Geometry check sheet. Reference: the model listing, model coordinates, mm. A direction names the side the tool comes from. Round coordinates to 2 decimals unless told otherwise and drop trailing zeros. Write each loop counter-clockwise with the first axis right and the second up, starting at its lowest first coordinate (ties: lowest second). Pieces come first, ordered by that corner, then holes. Notation, with made-up numbers: M 28,9.25 L 87,9.25 A24 cw 87,43.25 Z; hole C -27.75,84.5 d8. An arc over 180 degrees is marked long. Put each result on its own line as item: value. Start each with the question number.
(1) Section check B-B on y = -5.5. Record the cut outline in (x, z).
(2) Section check A-A on y = 1.25. Record the cut outline in (x, z), then the cut area to 3 significant figures.
(3) Tool access check on faces 1 (the conical face through (-0.2, -0.7, -8.92)), 2 (the cylindrical face through (-0.259, 6.108, -11.797)), 3 (the cylindrical face through (-0.1, -10.2, -6.8)). Record the directions out of +Z, -Z, +X, -X, +Y, -Y that give a thin tool (end or side, any length) a straight path to the whole face; none if there is none.
(4) Material ranges on probe 1 along Y at (x, z) = (-11, -1.25); probe 2 along X at (y, z) = (2, -4.5); probe 3 along X at (y, z) = (-2, -4.75), recorded low to high.
(5) Mould release check, pull along Y, two halves, no side actions. Record for faces 4 (the flat face through (0, 6.65, -12)), 5 (the conical face through (-0.2, 3.1, -10.8)), 6 (the conical face through (-0.13, -8.31, -5.76)): pulls with the +Y half, pulls with the -Y half, needs draft (parallel to the pull), parting line crosses it, or undercut.
(6) Gauge pin test, flat ends, axial feed: pin 1 (10 mm diameter, centred on x = 7, y = 2, fed in from -Z); pin 2 (6 mm diameter, centred on y = -6.5, z = -6.5, fed in from +X); pin 3 (1 mm diameter, centred on y = 1.5, z = -8, fed in from +X). Record the tip position at first contact, or that the pin passes through.
from build123d import *

# Parameters (mm, degrees)
F1_ANGLE     = 180
F2_T4_ANGLE  = 243.2500896942
F2_S5_R      = 11.8
F2_T6_DEPTH  = 16
F3_T4_ANGLE  = 243.6352501502
F3_S5_R      = 11.8
F3_T6_DEPTH  = 16
F4_T4_ANGLE  = 309.1355997924
F4_S5_R      = 6.8
F4_T6_DEPTH  = 11
F4_T10_ANGLE = 243.2500896942
F4_S11_R     = 11.8
F4_T12_DEPTH = 16
F5_SIZE      = 0.75
F6_SIZE      = 1


# Not quite as in the source:
# - a fillet or chamfer that OpenCascade refuses, or shapes differently, is made with other operations: its cross-section is extruded or revolved along the edge and cut away or added
# - a feature names something its author has since deleted; it is built from what else it names


with BuildPart() as f1:
    # F0 (on Top) → F1 (revolve)
    with BuildSketch(Plane.XY):
        Polygon((-11.8, 5.65), (-11.8, 6.65), (-13.8, 6.65), (-13.8, 0), (-7.8, -10.95), (-6.8, -10.95), (-6.8, -9.45), (-4.8, -9.45), (-4.8, -7.45), (-9.8, 1), (-11.8, 1), (-11.8, 2), (-9.8, 2), (-9.8, 5.65), align=None)
    revolve(axis=Axis((0, 0, 0), (0, -1, 0)), revolution_arc=F1_ANGLE)

    # F2: chamfer of 2.1 on 1 edges, made by hand


with BuildPart() as f2_tool2:
    # F2_s3 → F2_t4 (revolve)
    with BuildSketch(Plane(origin=(0, 0, 0), x_dir=(0, 1, 0), z_dir=(0.5243581586, 0, 0.8514978107))):
        Polygon((3.55, 9.8), (5.65, 11.9), (5.65, 9.8), align=None)
    revolve(axis=Axis((0, 5.65, 0), (0, -1, 0)), revolution_arc=F2_T4_ANGLE)

    # F2_s5 → F2_t6 (intersect, symmetric)
    with BuildSketch(Plane.XZ.offset(-4.6)):
        Circle(F2_S5_R)
    extrude(amount=F2_T6_DEPTH, both=True, mode=Mode.INTERSECT)


with BuildPart() as f1_1:
    add(f1.part)

    # F2_t1: cut F2_tool2
    add(f2_tool2.part, mode=Mode.SUBTRACT)

    # F3: chamfer of 2.1 on 1 edges, made by hand


with BuildPart() as f3_tool2:
    # F3_s3 → F3_t4 (revolve)
    with BuildSketch(Plane(origin=(0, 0, 0), x_dir=(0, 1, 0), z_dir=(0.5272172108, 0, 0.849730553))):
        Polygon((-0.8073066866, 8.7305877594), (1, 11.9), (1, 9.8), align=None)
    revolve(axis=Axis((0, 1, 0), (0, -1, 0)), revolution_arc=F3_T4_ANGLE)

    # F3_s5 → F3_t6 (intersect, symmetric)
    with BuildSketch(Plane.XZ.offset(-0.1)):
        Circle(F3_S5_R)
    extrude(amount=F3_T6_DEPTH, both=True, mode=Mode.INTERSECT)


with BuildPart() as f1_2:
    add(f1_1.part)

    # F3_t1: cut F3_tool2
    add(f3_tool2.part, mode=Mode.SUBTRACT)

    # F4: chamfer of 2.1 on 2 edges, made by hand


with BuildPart() as f4_tool2:
    # F4_s3 → F4_t4 (revolve)
    with BuildSketch(Plane(origin=(0, 0, 0), x_dir=(0, 1, 0), z_dir=(0.9030940896, 0, 0.4294427381))):
        Polygon((-7.35, 4.8), (-9.45, 6.9), (-9.45, 4.8), align=None)
    revolve(axis=Axis((0, -9.45, 0), (0, -1, 0)), revolution_arc=F4_T4_ANGLE)

    # F4_s5 → F4_t6 (intersect, symmetric)
    with BuildSketch(Plane.XZ.offset(8.4)):
        Circle(F4_S5_R)
    extrude(amount=F4_T6_DEPTH, both=True, mode=Mode.INTERSECT)


with BuildPart() as f1_3:
    add(f1_2.part)

    # F4_t1: cut F4_tool2
    add(f4_tool2.part, mode=Mode.SUBTRACT)


with BuildPart() as f4_tool8:
    # F4_s9 → F4_t10 (revolve)
    with BuildSketch(Plane(origin=(0, 0, 0), x_dir=(0, 1, 0), z_dir=(0.5243581586, 0, 0.8514978107))):
        Polygon((4.1, 9.8), (2, 11.9), (2, 9.8), align=None)
    revolve(axis=Axis((0, 2, 0), (0, -1, 0)), revolution_arc=F4_T10_ANGLE)

    # F4_s11 → F4_t12 (intersect, symmetric)
    with BuildSketch(Plane.XZ.offset(-3)):
        Circle(F4_S11_R)
    extrude(amount=F4_T12_DEPTH, both=True, mode=Mode.INTERSECT)


with BuildPart() as f1_4:
    add(f1_3.part)

    # F4_t7: cut F4_tool8
    add(f4_tool8.part, mode=Mode.SUBTRACT)

    # F5
    f5_edges = [f1_4.edges().sort_by_distance(p)[0] for p in [
        (0, 3.825, -10.075),
    ]]
    chamfer(f5_edges, length=F5_SIZE)

    # F6
    f6_edges = [f1_4.edges().sort_by_distance(p)[0] for p in [
        (0, -7.387175, -4.837175),
    ]]
    chamfer(f6_edges, length=F6_SIZE)


solid = f1_4.part
Answers follow:
1. outline: M -10.79,0 A10.79 ccw 10.79,0 L 5.95,0 A5.95 cw -5.95,0 Z
2. outline: M -13.8,0 A13.8 ccw 13.8,0 L 11.8,0 A11.8 cw -11.8,0 Z
2. area: 80.4 mm^2
3. face 1: +Z
3. face 2: +Z, +Y
3. face 3: +Z, -Y
4. probe 1: y = -4.98 to 0.53, 2.83 to 4.82
4. probe 2: x = -13.05 to -10.91, 10.91 to 13.05
4. probe 3: x = -11.78 to -6.47, 6.47 to 11.78
5. face 4: pulls with the +Y half
5. face 5: undercut
5. face 6: pulls with the -Y half
6. pin 1: stops at z = -13.65
6. pin 2: stops at x = 10.55
6. pin 3: stops at x = 11.58
